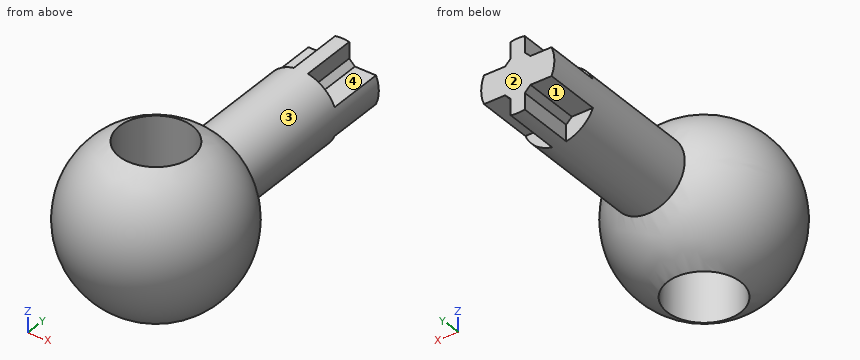
from build123d import *

# Parameters (mm, degrees)
SKETCH_S2_R              = 6.5
EXTRUDE_2_DEPTH          = 45
CUT_EXTRUDE_3_DEPTH      = 10
CHAMFER_4_SIZE           = 1
SKETCH_S5_R              = 6.5
CUT_EXTRUDE_5_DEPTH      = 16
CUT_EXTRUDE_5_DEPTH_BACK = 16


with BuildPart() as part:
    # Sketch s1 → Revolve 1 (revolve)
    with BuildSketch(Plane.XY):
        with BuildLine():
            Line((-15, 0), (15, 0))
            ThreePointArc((15, 0), (0, 15), (-15, 0))
        make_face()
    revolve(axis=Axis((-56.6721202, 0, 0), (1, 0, 0)))

    # Sketch s2 → Extrude 2 (add)
    with BuildSketch(Plane(origin=(0, 0, 0), x_dir=(1, 0, 0), z_dir=(0, 1, 0))):
        Circle(SKETCH_S2_R)
    extrude(amount=EXTRUDE_2_DEPTH)

    # Sketch s3 → Cut-Extrude 3 (cut)
    with BuildSketch(Plane(origin=(0, 45, 0), x_dir=(-1, 0, 0), z_dir=(0, 1, 0))):
        with BuildLine():
            Line((-1.25, -6.378675411), (-1.25, -2.5))
            Line((-1.25, -2.5), (-6, -2.5))
            ThreePointArc((-6, -2.5), (-4.111162334, -5.034713921), (-1.25, -6.378675411))
        make_face()
        with BuildLine():
            Line((1.25, -6.378675411), (1.25, -2.5))
            Line((1.25, -2.5), (6, -2.5))
            ThreePointArc((6, -2.5), (4.111162334, -5.034713921), (1.25, -6.378675411))
        make_face()
        with BuildLine():
            Line((-6, 2.5), (-1.25, 2.5))
            Line((-1.25, 2.5), (-1.25, 6.378675411))
            ThreePointArc((-1.25, 6.378675411), (-4.111162334, 5.034713921), (-6, 2.5))
        make_face()
        with BuildLine():
            Line((1.25, 2.5), (1.25, 6.378675411))
            ThreePointArc((1.25, 6.378675411), (4.111162334, 5.034713921), (6, 2.5))
            Line((6, 2.5), (1.25, 2.5))
        make_face()
    extrude(amount=-CUT_EXTRUDE_3_DEPTH, mode=Mode.SUBTRACT)

    # Chamfer 4
    chamfer_4_edges = [part.edges().sort_by_distance(p)[0] for p in [
        (-1.25, 40, -2.5),
        (-1.25, 40, 2.5),
        (1.25, 40, -2.5),
        (1.25, 40, 2.5),
    ]]
    chamfer(chamfer_4_edges, length=CHAMFER_4_SIZE)

    # Sketch s5 → Cut-Extrude 5 (cut, two sides)
    with BuildSketch(Plane.XY) as cut_extrude_5_sk:
        Circle(SKETCH_S5_R)
    extrude(amount=CUT_EXTRUDE_5_DEPTH, mode=Mode.SUBTRACT)
    extrude(cut_extrude_5_sk.sketch, amount=-CUT_EXTRUDE_5_DEPTH_BACK, mode=Mode.SUBTRACT)


solid = part.part
Work out the finished part from the listing and answer in its coordinate system (mm). Face numbers are marked on the shaded views. Give positions to 0.01 mm unless a question says otherwise; leave off trailing zeros. Write each loop counter-clockwise with the first axis right and the second up, starting at its lowest first coordinate (ties: lowest second). Pieces come first, ordered by that corner, then holes. Notation, with made-up numbers: (-24, 20) - (23, 20) arc R13 cw to (23, 35) - close; hole circle Ø8 at (16.5, 13). An arc over 180 degrees is marked (long way). One line per item, written item: value. Start each with the question number.
1. Consider probe 1 along X at (y, z) = (4.5, -9); probe 2 along Y at (x, z) = (0, -7.25); probe 3 along Y at (x, z) = (0, 6.75). Determine where each line is inside the solid, lowest interval first.
2. Find section A-A (x = 0). Write down the section's boundary in (y, z).
3. Find section D-D (y = 21). Write down the section's boundary in (x, z), then the cut area to 3 significant figures.
4. Find section C-C (z = 1.5). Write down the section's boundary in (x, y), then the cut area to 3 significant figures.
5. Given pin 1 (3 mm diameter, centred on x = -3, y = 39.5, fed in from +Z); pin 2 (5 mm diameter, centred on y = 36, z = -7, fed in from -X); pin 3 (0.9 mm diameter, centred on y = 39, z = 5.5, fed in from -X), each flat-ended and moving along its own axis, determine where each tip first touches the part or whether it passes through.
6. For a pull along Z with two mould halves and no side action, classify the marked faces 1, 2, 3 and 4 as +Z half, -Z half, draft (parallel to the pull), parting line (faces both ways), or undercut.
7. Find section B-B (y = 0). Write down the section's boundary in (x, z).
Geometry results:
1. probe 1: -11.12 to -4.69, 4.69 to 11.12
1. probe 2: -13.13 to -6.5, 6.5 to 13.13
1. probe 3: -13.4 to -6.5, 6.5 to 13.4
2. outline: (-6.5, -13.52) - (-6.5, 13.52) arc R15 ccw to start; (6.5, -13.52) arc R15 ccw to (13.52, -6.5) - (45, -6.5) - (45, 6.5) - (13.52, 6.5) arc R15 ccw to (6.5, 13.52) - close
3. outline: circle Ø13 at (0, 0)
3. area: 133 mm2
4. outline: (-6.32, 13.52) arc R14.92 ccw (long way) to (6.32, 13.52) - (6.32, 45) - (-6.32, 45) - close; hole circle Ø13 at (0, 0)
4. area: 953 mm2
5. pin 1: z = 3.25
5. pin 2: x = -4.48
5. pin 3: x = -1.25
6. face 1: -Z half
6. face 2: draft
6. face 3: parting line
6. face 4: +Z half
7. outline: (-6.5, -13.52) - (-6.5, 13.52) arc R15 ccw to start; (6.5, -13.52) arc R15 ccw to (6.5, 13.52) - close
